Model file for the job. Use its own axes, mm. A direction names the side the tool comes from. Give positions to 0.01 mm unless a question says otherwise; leave off trailing zeros. Loops run counter-clockwise (first coordinate to the right, second up) from the corner with the lowest first, then second, coordinate; pieces in that order, holes last. Notation, with made-up numbers: (73, 62.5) - (101, 62.5) arc R9 cw to (101, 75.5) - close; hole circle Ø10 at (19, 32). An arc over 180 degrees is marked (long way). Answer as CSV lines item,"result". Start each with the question number.
Item 1: Saw through at D-D on y = 8. Give the cut face in (x, z).
Item 2: Saw through at C-C on z = 12. Give the cut face in (x, y).
Item 3: Pull direction X, two halves, no side cores. Call faces 1 (the flat face through (-7, 7, -12)), 2 (the flat face through (-16.94, 18.92, 0.08)), 3 (the flat face through (2, 40, 6)): pulls with the +X half, pulls with the -X half, needs draft (parallel to the pull), parting line crosses it, or undercut.
Item 4: Pin check, flat tips, straight feed: pin 1 (12 mm diameter, centred on x = 19.5, y = 20, fed in from +Z); pin 2 (1 mm diameter, centred on x = -19, z = 12.5, fed in from +Y); pin 3 (2 mm diameter, centred on x = 21, z = -8.5, fed in from +Y); pin 4 (5.5 mm diameter, centred on x = -14.5, y = 16, fed in from -Z). Stop position of each tip, or through.
Item 5: Tool access for faces 4 (the flat face through (-9, 15, 13)), 5 (the flat face through (0, 45, -13.5)), 6 (the cylindrical face through (-1.172, 44.056, -8.923)), 7 (the flat face through (15, 14, -6)): list every direction of +Z, -Z, +X, -X, +Y, -Y with a clear straight run to the whole face (end or side of a thin tool).
Item 6: Drill centre lines: L1, parallel to Z at x = -20, y = 2.5; L2, parallel to Y at x = 0, z = 11.5; L3, parallel to X at y = 2, z = 12. Where is each one in solid material? Low to high. Write a range as from..to.
Item 7: Saw through at B-B on x = 0. Give the cut face in (y, z), plus the area to 3 significant figures.
Item 8: Saw through at A-A on y = 3. Give the cut face in (x, z).
from build123d import *

# Parameters (mm, degrees)
EXTRUDE_1_DEPTH          = 7
SKETCH_2_R               = 3
CUT_EXTRUDE_1_DEPTH      = 8
MIRROR_2_COPY_1_SKETCH_R = 3
MIRROR_2_COPY_1_DEPTH    = 8
SKETCH_3_R               = 13
EXTRUDE_2_DEPTH          = 35
EXTRUDE_3_DEPTH          = 6
SKETCH_5_R               = 9
CUT_EXTRUDE_2_DEPTH      = 8
SKETCH_6_R               = 6
CUT_EXTRUDE_3_DEPTH      = 41
EXTRUDE_4_REACH          = 36
CUT_EXTRUDE_4_REACH      = 36
SKETCH_8_R               = 6
EXTRUDE_5_DEPTH          = 6


with BuildPart() as part:
    # 草图1 → 凸台-拉伸1 (new body)
    with BuildSketch(Plane(origin=(0, 0, 0), x_dir=(1, 0, 0), z_dir=(0, 1, 0))):
        with BuildLine():
            Line((-27.110883423, 17), (27.110883423, 17))
            ThreePointArc((27.110883423, 17), (32, 0), (27.110883423, -17))
            Line((27.110883423, -17), (-27.110883423, -17))
            ThreePointArc((-27.110883423, -17), (-32, 0), (-27.110883423, 17))
        make_face()
    extrude(amount=EXTRUDE_1_DEPTH)

    # 草图2 → 切除-拉伸1 (cut, through all)
    with BuildSketch(Plane(origin=(0, 7, 0), x_dir=(1, 0, 0), z_dir=(0, 1, 0))):
        with Locations((-20, -12)):
            Circle(SKETCH_2_R)
    cut_extrude_1 = extrude(amount=-CUT_EXTRUDE_1_DEPTH, mode=Mode.SUBTRACT)

    # 镜向1: 切除-拉伸1 across plane
    add(cut_extrude_1.mirror(Plane(origin=(0, 0, 0), x_dir=(0, 0, 1), z_dir=(1, 0, 0))), mode=Mode.SUBTRACT)

    # 镜向2: 切除-拉伸1 across plane
    add(cut_extrude_1.mirror(Plane.XY), mode=Mode.SUBTRACT)

    # 镜向2 copy 1 sketch → 镜向2 copy 1 (cut, through all)
    with BuildSketch(Plane(origin=(0, 7, 0), x_dir=(-1, 0, 0), z_dir=(0, 1, 0))):
        with Locations((-20, -12)):
            Circle(MIRROR_2_COPY_1_SKETCH_R)
    extrude(amount=-MIRROR_2_COPY_1_DEPTH, mode=Mode.SUBTRACT)

    # 草图3 → 凸台-拉伸2 (add)
    with BuildSketch(Plane(origin=(0, 7, 0), x_dir=(1, 0, 0), z_dir=(0, 1, 0))):
        Circle(SKETCH_3_R)
    extrude(amount=EXTRUDE_2_DEPTH)

    # 草图4 → 凸台-拉伸3 (add)
    with BuildSketch(Plane(origin=(0, 42, 0), x_dir=(1, 0, 0), z_dir=(0, 1, 0))):
        with BuildLine():
            Line((-11.9058809, 13.5), (11.9058809, 13.5))
            ThreePointArc((11.9058809, 13.5), (18, 0), (11.9058809, -13.5))
            Line((11.9058809, -13.5), (-11.9058809, -13.5))
            ThreePointArc((-11.9058809, -13.5), (-18, 0), (-11.9058809, 13.5))
        make_face()
    extrude(amount=EXTRUDE_3_DEPTH)

    # 草图5 → 切除-拉伸2 (cut)
    with BuildSketch(Plane(origin=(0, 48, 0), x_dir=(1, 0, 0), z_dir=(0, 1, 0))):
        Circle(SKETCH_5_R)
    extrude(amount=-CUT_EXTRUDE_2_DEPTH, mode=Mode.SUBTRACT)

    # 草图6 → 切除-拉伸3 (cut, through all)
    with BuildSketch(Plane(origin=(0, 40, 0), x_dir=(1, 0, 0), z_dir=(0, 1, 0))):
        Circle(SKETCH_6_R)
    extrude(amount=-CUT_EXTRUDE_3_DEPTH, mode=Mode.SUBTRACT)

    # 草图7 → 凸台-拉伸4 (add, up to next)
    with BuildSketch(Plane.XY.offset(17), mode=Mode.PRIVATE) as extrude_4_sk1:
        with BuildLine():
            Line((-9, 23), (-9, 0))
            Line((-9, 0), (9, 0))
            Line((9, 0), (9, 23))
            ThreePointArc((9, 23), (0, 32), (-9, 23))
        make_face()
    extrude_4_tool1 = extrude(extrude_4_sk1.sketch, amount=-EXTRUDE_4_REACH, mode=Mode.PRIVATE) - part.part
    add(extrude_4_tool1.solids().sort_by_distance((0, 15.10139, 17))[0])

    # 草图8 → 切除-拉伸4 (cut, up to next)
    with BuildSketch(Plane.XY.offset(17), mode=Mode.PRIVATE) as cut_extrude_4_sk1:
        with Locations((0, 23)):
            Circle(SKETCH_8_R)
    cut_extrude_4_tool1 = extrude(cut_extrude_4_sk1.sketch, amount=-CUT_EXTRUDE_4_REACH, mode=Mode.PRIVATE) & part.part
    add(cut_extrude_4_tool1.solids().sort_by_distance((0, 23, 17))[0], mode=Mode.SUBTRACT)

    # 草图9 → 凸台-拉伸5 (add, symmetric)
    with BuildSketch(Plane.XY):
        Polygon((-22.5, 7), (-11.086673611, 7), (-11.086673611, 31.475957428), align=None)
    extrude_5 = extrude(amount=EXTRUDE_5_DEPTH, both=True)

    # 镜向3: 凸台-拉伸5 across plane
    add(extrude_5.mirror(Plane(origin=(0, 0, 0), x_dir=(0, 0, 1), z_dir=(1, 0, 0))))


solid = part.part
Responses:
1,outline,"(-22.03, -6) - (-11.53, -6) arc R13 ccw to (11.53, -6) - (22.03, -6) - (22.03, 6) - (11.53, 6) arc R13 ccw to (9, 9.38) - (9, 17) - (-9, 17) - (-9, 9.38) arc R13 ccw to (-11.53, 6) - (-22.03, 6) - close; hole circle Ø12 at (0, 0)"
2,outline,"(-29.66, 0) - (-23, 0) - (-23, 7) - (-29.66, 7) - close; (-17, 0) - (17, 0) - (17, 7) - (9, 7) - (9, 23) arc R9 ccw to (5, 30.48) - (5, 42) - (13.42, 42) - (13.42, 48) - (-13.42, 48) - (-13.42, 42) - (-5, 42) - (-5, 30.48) arc R9 ccw to (-9, 23) - (-9, 7) - (-17, 7) - close; (23, 0) - (29.66, 0) - (29.66, 7) - (23, 7) - close; hole circle Ø12 at (0, 23)"
3,face 1,"needs draft"
3,face 2,"pulls with the -X half"
3,face 3,"undercut"
4,pin 1,"z = 6"
4,pin 2,"through"
4,pin 3,"y = 7"
4,pin 4,"z = -6"
5,face 4,"+Z, -X"
5,face 5,"-Z, +X, -X, +Y"
5,face 6,"+Y"
5,face 7,"-Z, +X"
6,L1,"-17..-15, -9..9, 15..17"
6,L2,"0..17, 29..48"
6,L3,"-29.66..-23, -17..17, 23..29.66"
7,outline,"(0, -17) - (7, -17) - (7, -13) - (42, -13) - (42, -13.5) - (48, -13.5) - (48, -9) - (40, -9) - (40, -6) - (0, -6) - close; (0, 6) - (17, 6) - (17, 17) - (0, 17) - close; (29, 6) - (40, 6) - (40, 9) - (48, 9) - (48, 13.5) - (42, 13.5) - (42, 13) - (32, 13) - (32, 17) - (29, 17) - close"
7,area,"654 mm2"
8,outline,"(-27.11, -17) - (27.11, -17) arc R32 ccw to (27.11, 17) - (-27.11, 17) arc R32 ccw to start; hole circle Ø6 at (-20, -12); hole circle Ø6 at (-20, 12); hole circle Ø12 at (0, 0); hole circle Ø6 at (20, -12); hole circle Ø6 at (20, 12)"
